from build123d import *

# Parameters (mm, degrees)
CROQUIS1_W              = 4.8
CROQUIS1_H              = 2.4
CROQUIS1_W_2            = 22.5
CROQUIS1_H_2            = 23.8
SALIENTE_EXTRUIR1_DEPTH = 6.2
SALIENTE_EXTRUIR2_DEPTH = 4.2
CORTAR_EXTRUIR1_REACH   = 21.5
CORTAR_EXTRUIR3_DEPTH   = 0.8
CROQUIS4_5_W            = 1.5
CROQUIS4_5_H            = 3.75
CORTAR_EXTRUIR4_DEPTH   = 2
CORTAR_EXTRUIR5_DEPTH   = 13.4
CROQUIS7_R              = 2.425
CROQUIS7_R_2            = 0.875
SALIENTE_EXTRUIR4_DEPTH = 2.85
SKETCH1_R               = 6
BOSS_EXTRUDE1_DEPTH     = 50


with BuildPart() as part:
    # Croquis1 → Saliente-Extruir1 (new body, symmetric)
    with BuildSketch(Plane.XY):
        with Locations((-13.65, 6.4)):
            Rectangle(CROQUIS1_W, CROQUIS1_H)
        Rectangle(CROQUIS1_W_2, CROQUIS1_H_2)
        with Locations((13.65, 6.4)):
            Rectangle(CROQUIS1_W, CROQUIS1_H)
    extrude(amount=SALIENTE_EXTRUIR1_DEPTH, both=True)

    # Croquis2 → Saliente-Extruir2 (add)
    with BuildSketch(Plane(origin=(0, 11.9, 0), x_dir=(1, 0, 0), z_dir=(0, 1, 0))):
        with BuildLine():
            ThreePointArc((-0.484210526, -2.79508745), (11.25, 0), (-0.484210526, 2.79508745))
            ThreePointArc((-0.484210526, 2.79508745), (-3.45, 0), (-0.484210526, -2.79508745))
        make_face()
    extrude(amount=SALIENTE_EXTRUIR2_DEPTH)

    # Croquis3 → Cortar-Extruir1 (cut, up to next)
    with BuildSketch(Plane(origin=(0, 7.6, 0), x_dir=(1, 0, 0), z_dir=(0, 1, 0)), mode=Mode.PRIVATE) as cortar_extruir1_sk1:
        with BuildLine():
            Line((16.05, 0.575), (14.815922382, 0.575))
            ThreePointArc((14.815922382, 0.575), (12.35, 0), (14.815922382, -0.575))
            Line((14.815922382, -0.575), (16.05, -0.575))
            Line((16.05, -0.575), (16.05, 0.575))
        make_face()
    cortar_extruir1_tool1 = extrude(cortar_extruir1_sk1.sketch, amount=-CORTAR_EXTRUIR1_REACH, mode=Mode.PRIVATE) & part.part
    add(cortar_extruir1_tool1.solids().sort_by_distance((14.012834, 7.6, 0))[0], mode=Mode.SUBTRACT)
    # Croquis3 → Cortar-Extruir1 (cut, up to next)
    with BuildSketch(Plane(origin=(0, 7.6, 0), x_dir=(1, 0, 0), z_dir=(0, 1, 0)), mode=Mode.PRIVATE) as cortar_extruir1_sk2:
        with BuildLine():
            Line((-16.05, 0.575), (-14.815922382, 0.575))
            ThreePointArc((-14.815922382, 0.575), (-12.35, 0), (-14.815922382, -0.575))
            Line((-14.815922382, -0.575), (-16.05, -0.575))
            Line((-16.05, -0.575), (-16.05, 0.575))
        make_face()
    cortar_extruir1_tool2 = extrude(cortar_extruir1_sk2.sketch, amount=-CORTAR_EXTRUIR1_REACH, mode=Mode.PRIVATE) & part.part
    add(cortar_extruir1_tool2.solids().sort_by_distance((-14.012834, 7.6, 0))[0], mode=Mode.SUBTRACT)

    # Croquis4 → Cortar-Extruir3 (cut)
    with BuildSketch(Plane.XZ.offset(11.9)):
        with BuildLine():
            Line((-11.25, 6.2), (-11.25, 3.3))
            ThreePointArc((-11.25, 3.3), (-9.199390335, 4.149390335), (-8.35, 6.2))
            Line((-8.35, 6.2), (-11.25, 6.2))
        make_face()
        with BuildLine():
            ThreePointArc((-8.35, -6.2), (-9.199390335, -4.149390335), (-11.25, -3.3))
            Line((-11.25, -3.3), (-11.25, -6.2))
            Line((-11.25, -6.2), (-8.35, -6.2))
        make_face()
    extrude(amount=-CORTAR_EXTRUIR3_DEPTH, mode=Mode.SUBTRACT)

    # Croquis4_5 → Cortar-Extruir4 (cut)
    with BuildSketch(Plane.XZ.offset(11.9)):
        with BuildLine():
            Line((11.25, 6.2), (8.35, 6.2))
            ThreePointArc((8.35, 6.2), (9.199390335, 4.149390335), (11.25, 3.3))
            Line((11.25, 3.3), (11.25, 6.2))
        make_face()
        with BuildLine():
            ThreePointArc((11.25, -3.3), (9.199390335, -4.149390335), (8.35, -6.2))
            Line((8.35, -6.2), (11.25, -6.2))
            Line((11.25, -6.2), (11.25, -3.3))
        make_face()
        with Locations((10.5, 0)):
            Rectangle(CROQUIS4_5_W, CROQUIS4_5_H)
    extrude(amount=-CORTAR_EXTRUIR4_DEPTH, mode=Mode.SUBTRACT)

    # Croquis6 → Cortar-Extruir5 (cut, through all)
    with BuildSketch(Plane(origin=(0, 0, -6.2), x_dir=(-1, 0, 0), z_dir=(0, 0, -1))):
        Polygon((-11.25, -9.9), (-8.35, -11.9), (-11.25, -11.9), align=None)
    extrude(amount=-CORTAR_EXTRUIR5_DEPTH, mode=Mode.SUBTRACT)

    # Croquis7 → Saliente-Extruir4 (add)
    with BuildSketch(Plane(origin=(0, 16.1, 0), x_dir=(1, 0, 0), z_dir=(0, 1, 0))):
        with Locations((5.05, 0)):
            Circle(CROQUIS7_R)
        with Locations((5.05, 0)):
            Circle(CROQUIS7_R_2, mode=Mode.SUBTRACT)
    extrude(amount=SALIENTE_EXTRUIR4_DEPTH)

    # Sketch1 → Boss-Extrude1 (add)
    with BuildSketch(Plane(origin=(0, 18.95, 0), x_dir=(1, 0, 0), z_dir=(0, 1, 0))):
        with Locations((5.05, 0)):
            Circle(SKETCH1_R)
    extrude(amount=BOSS_EXTRUDE1_DEPTH)


solid = part.part
Could you check a few things on this model? Use its own coordinates, in mm. A direction names the side the tool comes from. Coordinates: 2 decimals unless noted, no trailing zeros. Order: outer loops, then holes, each group sorted by start corner. A loop starts at its lowest first (then second) coordinate and runs counter-clockwise, first axis right, second up.
Q1. Will these pins go through, and if not, where does the flat tip stop? pin 1 (3 mm diameter, centred on x = 0, y = 40.5, fed in from +Z); pin 2 (2.5 mm diameter, centred on x = -14, z = -3, fed in from -Y); pin 3 (6 mm diameter, centred on x = -7, z = 0, fed in from +Y).
Q2. Please list where these lines run through material, in increasing order: L1, parallel to X at y = 17.45, z = 0 (3 decimals); L2, parallel to Z at x = -13.65, y = 7.1; L3, parallel to Y at x = -0.5, z = 1.25.
Q3. Suppose I cut it at D-D on z = 4.25. Please give me the cut outline in (x, y).
Q4. Suppose I cut it at B-B on z = -4.5. Please give me the cut outline in (x, y), and give its area (3 significant figures).
Q5. Suppose I cut it at A-A on x = 13.65. Please give me the cut outline in (y, z), and give its area (3 significant figures).
Q6. Suppose I cut it at C-C on y = 56. Please give me the cut outline in (x, z), and give its area (3 significant figures).
Q7. Thinking about a two-plate mould opening in Z: for faces 4 (the cylindrical face through (12.35, 6.42, -0.05)), 5 (the cylindrical face through (5.885, 17.505, -0.263)), 6 (the cylindrical face through (8.86, -10.69, 4.56)), 7 (the flat face through (10, -9.9, -5)), which applies, released by +Z, released by -Z, zero draft, split by the parting line, or undercut?
Q8. Which directions (+Z, -Z, +X, -X, +Y, -Y) give clear straight access to the entire face, cutting with the end or side of a thin tool? Please do faces 1 (the flat face through (-5, 11.9, 0)), 2 (the cylindrical face through (-9.18, -11.51, -4.17)), 3 (the cylindrical face through (7.3, 17.5, 0.9)).
Answer:
1. pin 1: stops at z = 4.84
1. pin 2: stops at y = 5.2
1. pin 3: stops at y = 11.9
2. L1: x = 2.625 to 4.175, 5.925 to 7.475
2. L2: z = -6.2 to -1.3, 1.3 to 6.2
2. L3: y = -11.9 to 16.1, 18.95 to 68.95
3. outline: (-16.05, 5.2) - (-11.25, 5.2) - (-11.25, -11.1) - (-9.1, -11.1) - (-9.1, -11.9) - (8.35, -11.9) - (9.1, -11.38) - (9.1, -9.9) - (11.25, -9.9) - (11.25, 5.2) - (16.05, 5.2) - (16.05, 7.6) - (11.25, 7.6) - (11.25, 11.9) - (9.56, 11.9) - (9.56, 16.1) - (0.54, 16.1) - (0.54, 11.9) - (-11.25, 11.9) - (-11.25, 7.6) - (-16.05, 7.6) - close; (0.81, 18.95) - (9.29, 18.95) - (9.29, 68.95) - (0.81, 68.95) - close
4. outline: (-16.05, 5.2) - (-11.25, 5.2) - (-11.25, -11.1) - (-8.9, -11.1) - (-8.9, -11.9) - (8.35, -11.9) - (8.9, -11.52) - (8.9, -9.9) - (11.25, -9.9) - (11.25, 5.2) - (16.05, 5.2) - (16.05, 7.6) - (11.25, 7.6) - (11.25, 11.9) - (9.31, 11.9) - (9.31, 16.1) - (0.79, 16.1) - (0.79, 11.9) - (-11.25, 11.9) - (-11.25, 7.6) - (-16.05, 7.6) - close; (1.08, 18.95) - (9.02, 18.95) - (9.02, 68.95) - (1.08, 68.95) - close
4. area: 985 mm2
5. outline: (5.2, -6.2) - (7.6, -6.2) - (7.6, -1.3) - (5.2, -1.3) - close; (5.2, 1.3) - (7.6, 1.3) - (7.6, 6.2) - (5.2, 6.2) - close
5. area: 23.5 mm2
6. outline: circle Ø12 at (5.05, 0)
6. area: 113 mm2
7. face 4: undercut
7. face 5: undercut
7. face 6: released by +Z
7. face 7: zero draft
8. face 1: -X, +Y
8. face 2: -Z, -X, -Y
8. face 3: none
